The model under review builds one solid part; all positions refer to its coordinate system, in mm. A direction names the side the tool comes from. Give positions to 0.01 mm unless a question says otherwise; leave off trailing zeros. Order: outer loops, then holes, each group sorted by start corner. A loop starts at its lowest first (then second) coordinate and runs counter-clockwise, first axis right, second up. Notation, with made-up numbers: (15.25, -23.75) - (61.25, -23.75) arc R20 cw to (61.25, 15.25) - close; hole circle Ø4 at (-31, -34). An arc over 180 degrees is marked (long way). Use CSV: the item, a comma, the result in double quotes. Start each with the question number.
```python
from build123d import *

# Parameters (mm, degrees)
SKETCH1_R           = 114.3
SKETCH1_R_2         = 1.1303
SKETCH1_R_3         = 105
BOSS_EXTRUDE1_DEPTH = 0.254
BOSS_EXTRUDE2_START = -20
BOSS_EXTRUDE2_DEPTH = 20
CUT_EXTRUDE1_DEPTH  = 268.813456051
CIRPATTERN1_COUNT   = 2


with BuildPart() as part:
    # Sketch1 → Boss-Extrude1 (new body)
    # profile 1 of 2: a face of its own
    with BuildSketch(Plane.XY):
        with Locations((-20.073709177, -8.103148659)):
            Circle(SKETCH1_R)
        with Locations((-113.658579374, -62.134398659)):
            Circle(SKETCH1_R_2, mode=Mode.SUBTRACT)
        with Locations((-20.073709177, -116.165648659)):
            Circle(SKETCH1_R_2, mode=Mode.SUBTRACT)
        with Locations((73.511161019, -62.134398659)):
            Circle(SKETCH1_R_2, mode=Mode.SUBTRACT)
        with Locations((73.511161019, 45.928101341)):
            Circle(SKETCH1_R_2, mode=Mode.SUBTRACT)
        with Locations((-20.073709177, 99.959351341)):
            Circle(SKETCH1_R_2, mode=Mode.SUBTRACT)
        with Locations((-20.073709177, -8.103148659)):
            Circle(SKETCH1_R_3, mode=Mode.SUBTRACT)
        with Locations((-113.658579374, 45.928101341)):
            Circle(SKETCH1_R_2, mode=Mode.SUBTRACT)
    # profile 2 of 2: a face of its own
    with BuildSketch(Plane.XY):
        with Locations((-20.073709177, -8.103148659)):
            Circle(SKETCH1_R_3)
    extrude(amount=BOSS_EXTRUDE1_DEPTH)

    # Sketch2 → Boss-Extrude2 (add)
    with BuildSketch(Plane.XY.offset(0.254).offset(BOSS_EXTRUDE2_START)):
        with BuildLine():
            Line((3.743406653, 103.947571596), (3.690597083, 103.699122105))
            ThreePointArc((3.690597083, 103.699122105), (9.509307678, 102.302173286), (15.24693328, 100.602611154))
            Line((15.24693328, 100.602611154), (15.325423596, 100.844179509))
            ThreePointArc((15.325423596, 100.844179509), (9.575047716, 102.547518446), (3.743406653, 103.947571596))
        make_face()
    boss_extrude2 = extrude(amount=BOSS_EXTRUDE2_DEPTH)

    # Sketch3 → Cut-Extrude1 (cut, through all)
    with BuildSketch(Plane(origin=(9.575047716, 102.547518446, 0.254), x_dir=(-0.96592582628907, 0.25881904510251436, 0), z_dir=(0.25881904510251436, 0.96592582628907, 0))):
        with BuildLine():
            ThreePointArc((0, -8.62205), (-1.63195, -10.254), (0, -11.88595))
            Line((0, -11.88595), (0, -8.62205))
        make_face()
        with BuildLine():
            Line((0, -8.62205), (0, -11.88595))
            ThreePointArc((0, -11.88595), (1.153962912, -11.407962912), (1.63195, -10.254))
            ThreePointArc((1.63195, -10.254), (1.153962912, -9.100037088), (0, -8.62205))
        make_face()
        with BuildLine():
            ThreePointArc((5.995293131, -15), (4.530827037, -18.535533906), (0.995293131, -20))
            Line((0.995293131, -20), (5.995293131, -20))
            Line((5.995293131, -20), (5.995293131, -15))
        make_face()
        with BuildLine():
            Line((-5.995293131, -20), (-0.995293131, -20))
            ThreePointArc((-0.995293131, -20), (-4.530827037, -18.535533906), (-5.995293131, -15))
            Line((-5.995293131, -15), (-5.995293131, -20))
        make_face()
    cut_extrude1 = extrude(amount=-CUT_EXTRUDE1_DEPTH, mode=Mode.SUBTRACT)

    # CirPattern1: Boss-Extrude2, Cut-Extrude1 ×2 about axis
    cirpattern1_axis = Axis((-20.073709177, -8.103148659, 0), (0, 0, 1))
    add([boss_extrude2.rotate(cirpattern1_axis, i * 360 / CIRPATTERN1_COUNT) for i in range(1, CIRPATTERN1_COUNT)])
    add([cut_extrude1.rotate(cirpattern1_axis, i * 360 / CIRPATTERN1_COUNT) for i in range(1, CIRPATTERN1_COUNT)], mode=Mode.SUBTRACT)


solid = part.part
```
1. Tool access review of faces 1 (the face through (-49.58, -118.53, -7.82)), 2 (the face through (9.428, 102.324, -7.817)), 3 (the face through (-49.804, -118.732, -7.664)): name each direction out of +Z, -Z, +X, -X, +Y, -Y from which nothing blocks a thin tool from reaching the whole face with its end or side.
2. Consider section B-B (x = -41). Give the boundary of the cut face in (y, z).
3. Clearance check with flat-ended pins moving along their axes: pin 1 (10 mm diameter, centred on x = -33, z = -8, fed in from -Y); pin 2 (12 mm diameter, centred on y = 29.5, z = -3.5, fed in from -X); pin 3 (2.5 mm diameter, centred on x = 73.51, y = -62.13, fed in from -Z). State where each tip first meets the part, or that it passes through.
4. To check wall thickness, follow L1, parallel to Z at x = 16.5, y = -52; L2, parallel to Y at x = -49.5, z = -12.25. State the ranges of each line that lie inside material, in increasing order. Write a range as [from, to].
5. Consider section A-A (y = -96). Give the boundary of the cut face in (x, z), and give its area (3 significant figures).
Answers follow:
1,face 1,"-Z, +X, +Y"
1,face 2,"-Z, -X, -Y"
1,face 3,"+Z, -Z, -X, -Y"
2,outline,"(-120.47, 0) - (104.26, 0) - (104.26, 0.25) - (-120.47, 0.25) - close"
3,pin 1,"passes through"
3,pin 2,"stops at x = -129.59"
3,pin 3,"stops at z = 0"
4,L1,"z = [0, 0.25]"
4,L2,"y = [-118.81, -118.55]"
5,outline,"(-93.14, 0) - (52.99, 0) - (52.99, 0.25) - (-93.14, 0.25) - close"
5,area,"37.1 mm^2"
